Verification items for the finished model (mm, model axes). A direction names the side the tool comes from. Give positions to 0.01 mm unless a question says otherwise; leave off trailing zeros. Order: outer loops, then holes, each group sorted by start corner. A loop starts at its lowest first (then second) coordinate and runs counter-clockwise, first axis right, second up. Notation, with made-up numbers: (54.25, -17.5) -> (108.25, -17.5) arc R16 cw to (108.25, -11.5) -> close; hole circle Ø3 at (23, 37). An arc over 180 degrees is marked (long way). Return JSON: item names as keys, results as strings. Group by question number.
(1) Cross-section at B-B on x = 28. Enter the section's corners in (y, z), then the cut area to 3 significant figures.
(2) Depth check by flat-ended pin: pin 1 Ø3 at (x, y) = (-11.5, -46.5) entering from -Z; pin 2 Ø7 at (x, y) = (-42.5, 32) entering from +Z; pin 3 Ø1.5 at (x, y) = (27.5, 33) entering from -Z; pin 4 Ø2 at (x, z) = (59.5, -13.5) entering from +Y. Enter the tip coordinate at first touch or a pass-through.
(3) Cross-section at A-A on y = 7. Enter the section's corners in (x, z), then the cut area to 3 significant figures.
(4) Release check for a two-part mould opening along Z. For faces 4 (the face through (20.235, -51.683, -11.022)), 5 (the face through (1.01, -50.79, -12.28)), 6 (the face through (53.79, -51.78, -11.14)), 7 (the face through (-41.7, 30.7, -1)) record: pulls with the +Z half, pulls with the -Z half, needs draft (parallel to the pull), parting line crosses it, or undercut.
(5) Cross-section at D-D on y = -40. Enter the section's corners in (x, z).
(6) Thickness scan on line 1 along X through (y, z) = (-4.5, -2); line 2 along Y through (x, z) = (53, -2.15); line 3 along Y through (x, z) = (43, -0.5). Record the ranges inside material, lowest first.
(7) Tool access check on faces 1 (the face through (-51.7, 30.7, -1)), 2 (the face through (-1, 1, -3)), 3 (the face through (-16.765, -51.683, -11.022)). Record the directions out of +Z, -Z, +X, -X, +Y, -Y that give a thin tool (end or side, any length) a straight path to the whole face; none if there is none.
(8) Cross-section at C-C on x = -2. Enter the section's corners in (y, z), then the cut area to 3 significant figures.
from build123d import *

# Parameters (mm, degrees)
SKETCH_2_W           = 214
SKETCH_2_H           = 90
EXTRUDE_5_DEPTH      = 3
SKETCH_14_R          = 1.55
CUT_EXTRUDE_12_DEPTH = 117.116320989
SKETCH_15_R          = 3.1
CUT_EXTRUDE_14_DEPTH = 1
SKETCH_11_W          = 48
SKETCH_11_H          = 48
CUT_EXTRUDE_15_DEPTH = 117.116320989
EXTRUDE_6_DEPTH      = 214
EXTRUDE_7_DEPTH      = 214
SKETCH_13_R          = 1.75
CUT_EXTRUDE_16_DEPTH = 134.72337904
SKETCH_23_W          = 35
SKETCH_23_H          = 23.89847847
CUT_EXTRUDE_17_DEPTH = 135.831639748
FILLET_3_R           = 3
FILLET_4_R           = 3


with BuildPart() as part:
    # 草图2 → 凸台-拉伸5 (new body)
    with BuildSketch(Plane.XY):
        Rectangle(SKETCH_2_W, SKETCH_2_H)
    extrude(amount=-EXTRUDE_5_DEPTH)

    # 草图14 → 切除-拉伸12 (cut, through all)
    with BuildSketch(Plane(origin=(0, 0, -3), x_dir=(-1, 0, 0), z_dir=(0, 0, -1))):
        with Locations((-53, 32)):
            Circle(SKETCH_14_R)
        with Locations((-43, 32)):
            Circle(SKETCH_14_R)
        with Locations((43, 32)):
            Circle(SKETCH_14_R)
        with Locations((53, 32)):
            Circle(SKETCH_14_R)
    extrude(amount=-CUT_EXTRUDE_12_DEPTH, mode=Mode.SUBTRACT)

    # 草图15 → 切除-拉伸14 (cut)
    with BuildSketch(Plane.XY):
        with Locations((53, 32)):
            Circle(SKETCH_15_R)
        with Locations((43, 32)):
            Circle(SKETCH_15_R)
        with Locations((-43, 32)):
            Circle(SKETCH_15_R)
        with Locations((-53, 32)):
            Circle(SKETCH_15_R)
    extrude(amount=-CUT_EXTRUDE_14_DEPTH, mode=Mode.SUBTRACT)

    # 草图11 → 切除-拉伸15 (cut, through all)
    with BuildSketch(Plane(origin=(0, 0, -3), x_dir=(-1, 0, 0), z_dir=(0, 0, -1))):
        with Locations((-34, -9)):
            Rectangle(SKETCH_11_W, SKETCH_11_H)
        with Locations((34, -9)):
            Rectangle(SKETCH_11_W, SKETCH_11_H)
    extrude(amount=-CUT_EXTRUDE_15_DEPTH, mode=Mode.SUBTRACT)

    # 草图21 → 凸台-拉伸6 (add, through all)
    with BuildSketch(Plane(origin=(107, 0, 0), x_dir=(0, 0, -1), z_dir=(1, 0, 0))):
        Polygon((0, -45), (19.987130176, -60.615657522), (21.124247333, -59.160213932), (3, -45), align=None)
    extrude(amount=-EXTRUDE_6_DEPTH)

    # 草图22 → 凸台-拉伸7 (add, through all)
    with BuildSketch(Plane(origin=(107, 0, 0), x_dir=(0, 0, -1), z_dir=(1, 0, 0))):
        Polygon((3, -43.540629053), (21.83225803, -58.254001566), (21.124247333, -59.160213932), (3, -45), align=None)
    extrude(amount=-EXTRUDE_7_DEPTH)

    # 草图13 → 切除-拉伸16 (cut, through all)
    with BuildSketch(Plane(origin=(0, -24.123766801, 18.847552259), x_dir=(1, 0, 0), z_dir=(0, 0.788010753606719, -0.615661475325662))):
        with Locations(Location((55.5, 40.277161152, 0), (0, 0, 270))):
            Circle(SKETCH_13_R)
        with Locations(Location((18.5, 40.277161152, 0), (0, 0, 270))):
            Circle(SKETCH_13_R)
        with Locations(Location((-18.5, 40.277161152, 0), (0, 0, 270))):
            Circle(SKETCH_13_R)
        with Locations(Location((-55.5, 40.277161152, 0), (0, 0, 270))):
            Circle(SKETCH_13_R)
    extrude(amount=-CUT_EXTRUDE_16_DEPTH, mode=Mode.SUBTRACT)

    # 草图23 → 切除-拉伸17 (cut, through all)
    with BuildSketch(Plane(origin=(0, -25.581586695, 19.986525988), x_dir=(1, 0, 0), z_dir=(0, 0.788010753606719, -0.6156614753256621))):
        with Locations((-89.5, 41.119559415)):
            Rectangle(SKETCH_23_W, SKETCH_23_H)
        with Locations((89.5, 41.119559415)):
            Rectangle(SKETCH_23_W, SKETCH_23_H)
    extrude(amount=-CUT_EXTRUDE_17_DEPTH, mode=Mode.SUBTRACT)

    # 圆角3
    fillet_3_edges = [part.edges().sort_by_distance(p)[0] for p in [
        (-107, 45, -1.5),
    ]]
    fillet(fillet_3_edges, radius=FILLET_3_R)

    # 圆角4
    fillet_4_edges = [part.edges().sort_by_distance(p)[0] for p in [
        (107, 45, -1.5),
    ]]
    fillet(fillet_4_edges, radius=FILLET_4_R)


solid = part.part
Verdict:
{
 "1": {"outline": "(-60.62, -19.99) -> (-58.25, -21.83) -> (-43.54, -3) -> (-33, -3) -> (-33, 0) -> (-45, 0) -> close; (15, -3) -> (45, -3) -> (45, 0) -> (15, 0) -> close", "area": "198 mm²"},
 "2": {"pin 1": "z = -8.71", "pin 2": "z = 0", "pin 3": "z = -3", "pin 4": "y = -50.96"},
 "3": {"outline": "(-107, -3) -> (-58, -3) -> (-58, 0) -> (-107, 0) -> close; (-10, -3) -> (10, -3) -> (10, 0) -> (-10, 0) -> close; (58, -3) -> (107, -3) -> (107, 0) -> (58, 0) -> close", "area": "354 mm²"},
 "4": {"face 4": "undercut", "face 5": "pulls with the -Z half", "face 6": "undercut", "face 7": "pulls with the +Z half"},
 "5": {"outline": "(-107, -3) -> (107, -3) -> (107, 0) -> (-107, 0) -> close"},
 "6": {"line 1": "-107 to -58, -10 to 10, 58 to 107", "line 2": "-46.68 to -33, 15 to 30.45, 33.55 to 45", "line 3": "-45.39 to -33, 15 to 28.9, 35.1 to 45"},
 "7": {"face 1": "+Z", "face 2": "-Z, +X, -X, +Y", "face 3": "none"},
 "8": {"outline": "(-60.62, -19.99) -> (-58.25, -21.83) -> (-43.54, -3) -> (45, -3) -> (45, 0) -> (-45, 0) -> close", "area": "342 mm²"}
}
